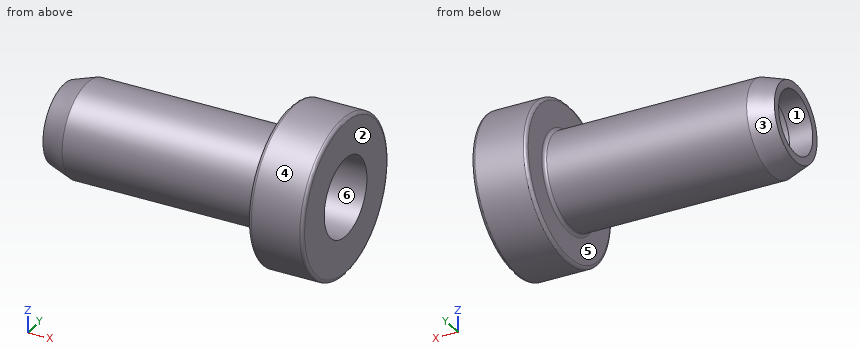
Autodesk Inventor part; units mm, degrees
ref_plane "YZ Plane" through (0, 0, 0) normal (1, 0, 0) x (0, 1, 0)
ref_plane "XZ Plane" through (0, 0, 0) normal (0, 1, 0) x (-1, 0, 0)
ref_plane "XY Plane" through (0, 0, 0) normal (0, 0, 1) x (1, 0, 0)
sketch "Skizze1" plane through (0, 0, 0) normal (0, 0, 1) x (1, 0, 0)
  line L0 (-16.5, 2.5) -> (0, 2.5)
  line L1 (0, 5) -> (-3.5, 5)
  line L2 (0, 5) -> (0, 2.5)
  line L3 (-3.5, 5) -> (-3.5, 3)
  line L4 (-3.5, 3) -> (-16.5, 3)
  line L5 (-18, 2.5) -> (-16.5, 3)
  line L6 (-16.5, 2) -> (-18, 2)
  line L7 (-16.5, 2) -> (-16.5, 2.5)
  line L8 (-18, 2.5) -> (-18, 2)
  line L9 (0, 1.4) -> (0, 5.6)
  line L10 (-21.6, 0) -> (3.6, 0)
  dimension "d0" = 5
  dimension "d1" = 10
  dimension "d2" = 6
  dimension "d3" = 1.5
  dimension "d4" = 4
  dimension "d5" = 18
  dimension "d6" = 3.5
  dimension "d7" = 161.565
revolve "Umdrehung1" add sketch "Skizze1" angle 360 about axis through (-10, 0, 0) along (1, 0, 0)
thread "Gewinde1"
fillet "Rundung1" radius 0.2 3 edges at (-3.5, -3, 0) (-3.5, -5, 0) (0, -5, 0)
properties part number "YTP-AP-E12-R1.0"
Geometry check sheet. Reference: the model listing, model coordinates, mm. Face numbers are marked on the shaded views. A direction names the side the tool comes from. Give positions to 0.01 mm unless a question says otherwise; leave off trailing zeros. Write each loop counter-clockwise with the first axis right and the second up, starting at its lowest first coordinate (ties: lowest second). Pieces come first, ordered by that corner, then holes. Notation, with made-up numbers: (3, 77) -> (29, 77) arc R18 ccw to (29, 105) -> close; hole circle Ø8 at (9.25, 89). An arc over 180 degrees is marked (long way). Use one line per item in the form item = value.
Item 1: Mould release check, pull along Z, two halves, no side actions. Record for the marked faces 1, 2 and 3: released by +Z, released by -Z, zero draft, split by the parting line, or undercut.
Results list:
face_1 = undercut
face_2 = zero draft
face_3 = split by the parting line
Item 2: Sectioned sample at D-D on x = -3. Enter the section's corners in (y, z).
Results list:
outline = circle Ø10 at (0, 0); hole circle Ø5 at (0, 0)
Item 3: Scan lines: line 1 (Z direction, x = -8, y = 0); line 2 (X direction, y = -1.75, z = 3.75); line 3 (Y direction, x = -12, z = 1.75). Record each from-to range of solid material in increasing order.
Results list:
line_1 = -3 to -2.5, 2.5 to 3
line_2 = -3.5 to 0
line_3 = -2.44 to -1.79, 1.79 to 2.44
Item 4: Depth check by flat-ended pin: pin 1 Ø4.5 at (y, z) = (0, 0) entering from +X; pin 2 Ø6 at (x, z) = (-10, 0.5) entering from -Y; pin 3 Ø1.5 at (y, z) = (0.5, 1) entering from +X; pin 4 Ø3 at (x, z) = (-8, -3.5) entering from +Y. Enter the tip coordinate at first touch or a pass-through.
Results list:
pin_1 = -16.5
pin_2 = -3
pin_3 = through
pin_4 = 2.24
Item 5: Sectioned sample at A-A on z = 0. Enter the section's corners in (x, y), plus the area to 3 significant figures.
Results list:
outline = (-18, -2.5) -> (-16.5, -3) -> (-3.7, -3) arc R0.2 cw to (-3.5, -3.2) -> (-3.5, -4.8) arc R0.2 ccw to (-3.3, -5) -> (-0.2, -5) arc R0.2 ccw to (0, -4.8) -> (0, -2.5) -> (-16.5, -2.5) -> (-16.5, -2) -> (-18, -2) -> close; (-18, 2) -> (-16.5, 2) -> (-16.5, 2.5) -> (0, 2.5) -> (0, 4.8) arc R0.2 ccw to (-0.2, 5) -> (-3.3, 5) arc R0.2 ccw to (-3.5, 4.8) -> (-3.5, 3.2) arc R0.2 cw to (-3.7, 3) -> (-16.5, 3) -> (-18, 2.5) -> close
area = 32.7 mm2
Item 6: Sectioned sample at C-C on x = -6. Enter the section's corners in (y, z), plus the area to 3 significant figures.
Results list:
outline = circle Ø6 at (0, 0); hole circle Ø5 at (0, 0)
area = 8.64 mm2
Item 7: Access from +Z, -Z, +X, -X, +Y, -Y to the whole of each face (thin tool, end or side, straight path). Record for the marked faces 4, 5 and 6.
Results list:
face_4 = +X, -X
face_5 = -X
face_6 = +X
